Design review of the part built by this model. Coordinates are the model's own, in mm. A direction names the side the tool comes from. Coordinates: 2 decimals unless noted, no trailing zeros. Loops run counter-clockwise (first coordinate to the right, second up) from the corner with the lowest first, then second, coordinate; pieces in that order, holes last. Notation, with made-up numbers: M 4,21 L 45,21 A8 cw 45,33 Z; hole C 37.5,74 d4. An arc over 180 degrees is marked long. Put each result on its own line as item: value. Start each with the question number.
(1) Take a section at A-A, the plane x = 36. Give the boundary of the cut face in (y, z), then the cut area to 3 significant figures.
(2) For probe 1 along Z at (x, y) = (-34, 3.05); probe 2 along Z at (x, y) = (20.5, 0.3); probe 3 along X at (y, z) = (2.15, 35), list the stretches that pass through material, from the lowest coordinate up. Write a range as [from, to].
(3) For faces 1 (the flat face through (-1, 5, 53)), 2 (the flat face through (-1, 2, -50)), 3 (the flat face through (-1, 3, 58)), list the 3-axis set-ups (+Z, -Z, +X, -X, +Y, -Y) from which the entire face can be reached by the end or side of a thin tool; tool diameter is ignored.
(4) Take a section at C-C, the plane x = 0. Give the boundary of the cut face in (y, z).
(5) Take a section at B-B, the plane z = -37.5. Give the boundary of the cut face in (x, y).
(6) Take a section at D-D, the plane y = 1.3. Give the boundary of the cut face in (x, z).
(7) The part is to be moulded in two halves that separate along X. For faces 4 (the flat face through (67, 3, -56)), 5 (the flat face through (50, 2, 1)), 6 (the flat face through (-68, 3, 1)), say which applies: +X half, -X half, draft (parallel to the pull), parting line (faces both ways), or undercut.
```python
from build123d import *

# Parameters (mm, degrees)
SKETCH_3_W          = 136
SKETCH_3_H          = 116
EXTRUDE_2_DEPTH     = 6
SKETCH_4_W          = 106
SKETCH_4_H          = 106
CUT_EXTRUDE_1_DEPTH = 3
SKETCH_5_W          = 100
SKETCH_5_H          = 100
CUT_EXTRUDE_2_DEPTH = 10
CHAMFER_1_SIZE      = 3
SKETCH_6_R          = 1.5
CUT_EXTRUDE_3_DEPTH = 10


with BuildPart() as part:
    # 스케치3 → 보스-돌출2 (new body)
    with BuildSketch(Plane(origin=(0, 0, 0), x_dir=(1, 0, 0), z_dir=(0, 1, 0))):
        Rectangle(SKETCH_3_W, SKETCH_3_H)
    extrude(amount=EXTRUDE_2_DEPTH)

    # 스케치4 → 컷-돌출1 (cut)
    with BuildSketch(Plane(origin=(0, 6, 0), x_dir=(1, 0, 0), z_dir=(0, 1, 0))):
        Rectangle(SKETCH_4_W, SKETCH_4_H)
    extrude(amount=-CUT_EXTRUDE_1_DEPTH, mode=Mode.SUBTRACT)

    # 스케치5 → 컷-돌출2 (cut)
    with BuildSketch(Plane(origin=(0, 3, 0), x_dir=(1, 0, 0), z_dir=(0, 1, 0))):
        Rectangle(SKETCH_5_W, SKETCH_5_H)
    extrude(amount=-CUT_EXTRUDE_2_DEPTH, mode=Mode.SUBTRACT)

    # 모따기1
    chamfer_1_edges = [part.edges().sort_by_distance(p)[0] for p in [
        (68, 3, 58),
        (-68, 3, 58),
        (-68, 3, -58),
        (68, 3, -58),
    ]]
    chamfer(chamfer_1_edges, length=CHAMFER_1_SIZE)

    # 스케치6 → 컷-돌출3 (cut)
    with BuildSketch(Plane(origin=(0, 6, 0), x_dir=(1, 0, 0), z_dir=(0, 1, 0))):
        with Locations(Location((0, 55.5, 0), (0, 0, 270))):
            Circle(SKETCH_6_R)
    extrude(amount=-CUT_EXTRUDE_3_DEPTH, mode=Mode.SUBTRACT)


solid = part.part
```
Computed values:
1. outline: M 0,-58 L 6,-58 L 6,-53 L 3,-53 L 3,-50 L 0,-50 Z; M 0,50 L 3,50 L 3,53 L 6,53 L 6,58 L 0,58 Z
1. area: 78.0 mm^2
2. probe 1: z = [-58, -53], [53, 58]
2. probe 2: z = [-58, -50], [50, 58]
2. probe 3: x = [-68, -50], [50, 68]
3. face 1: +Y
3. face 2: +Y, -Y
3. face 3: +Z, +X, -X, +Y, -Y
4. outline: M 0,-58 L 6,-58 L 6,-57 L 0,-57 Z; M 0,-54 L 6,-54 L 6,-53 L 3,-53 L 3,-50 L 0,-50 Z; M 0,50 L 3,50 L 3,53 L 6,53 L 6,58 L 0,58 Z
5. outline: M -68,0 L -50,0 L -50,3 L -53,3 L -53,6 L -68,6 Z; M 50,0 L 68,0 L 68,6 L 53,6 L 53,3 L 50,3 Z
6. outline: M -68,-55 L -65,-58 L 65,-58 L 68,-55 L 68,55 L 65,58 L -65,58 L -68,55 Z; hole M -50,-50 L 50,-50 L 50,50 L -50,50 Z; hole C 0,-55.5 d3
7. face 4: +X half
7. face 5: undercut
7. face 6: -X half
